The listing builds one solid part. Answer for the finished solid, in the listing's coordinates (mm). A direction names the side the tool comes from. Give positions to 0.01 mm unless a question says otherwise; leave off trailing zeros. Loops run counter-clockwise (first coordinate to the right, second up) from the corner with the lowest first, then second, coordinate; pieces in that order, holes last. Notation, with made-up numbers: (41.25, 85) - (91.25, 85) arc R29 cw to (91.25, 114) - close; hole circle Ø2 at (37.25, 14.5). An arc over 180 degrees is marked (long way). Write each question's results on one line, items separated by ' | '.
from build123d import *

# Parameters (mm, degrees)
SKETCH1_W                                            = 355
SKETCH1_H                                            = 188
BOSS_EXTRUDE1_DEPTH                                  = 3
EDGE_FLANGE1_STRIP_W                                 = 20
EDGE_FLANGE1_STRIP_H                                 = 3
EDGE_FLANGE1_STRIP_CUT_DEPTH                         = 188
EDGE_FLANGE1_DEPTH                                   = 188
SKETCH11_R                                           = 21.5
CUT_EXTRUDE2_DEPTH                                   = 10
CSK_FOR_M4_HEX_SOCKET_COUNTERSUNK_HEAD_S_D           = 4.5
CSK_FOR_M4_HEX_SOCKET_COUNTERSUNK_HEAD_S_DEPTH       = 10
CSK_FOR_M4_HEX_SOCKET_COUNTERSUNK_HEAD_S_CSINK_D     = 9.18
CSK_FOR_M4_HEX_SOCKET_COUNTERSUNK_HEAD_S_CSINK_ANGLE = 90
CSK_FOR_M4_HEX_SOCKET_COUNTERSUNK_HEAD_S_TIP         = 1.351936393
EDGE_FLANGE2_STRIP_W                                 = 20
EDGE_FLANGE2_STRIP_H                                 = 3
EDGE_FLANGE2_STRIP_CUT_DEPTH                         = 188
EDGE_FLANGE2_DEPTH                                   = 188
SKETCH19_W                                           = 210
SKETCH19_H                                           = 48
BOSS_EXTRUDE2_DEPTH                                  = 3
FILLET1_R                                            = 10
EDGE_FLANGE3_STRIP_W                                 = 20
EDGE_FLANGE3_STRIP_H                                 = 3
EDGE_FLANGE3_STRIP_CUT_DEPTH                         = 210
EDGE_FLANGE3_STRIP_2_W                               = 20
EDGE_FLANGE3_STRIP_2_H                               = 3
EDGE_FLANGE3_STRIP_CUT_2_DEPTH                       = 210
EDGE_FLANGE3_DEPTH                                   = 210
EDGE_FLANGE3_BEND_DEPTH                              = 210
SKETCH26_R                                           = 2.1
CUT_EXTRUDE3_DEPTH                                   = 10
SKETCH28_W                                           = 50
SKETCH28_H                                           = 30
CUT_EXTRUDE4_DEPTH                                   = 10
SKETCH29_W                                           = 87
SKETCH29_H                                           = 23.35234987
CUT_EXTRUDE5_DEPTH                                   = 10
FILLET2_R                                            = 10
SKETCH30_R                                           = 2.5
SKETCH30_R_2                                         = 1.57499812
CUT_EXTRUDE6_DEPTH                                   = 10
SKETCH31_R                                           = 2.1
CUT_EXTRUDE7_DEPTH                                   = 236
SKETCH32_R                                           = 2.5
CUT_EXTRUDE8_DEPTH                                   = 10
SKETCH33_R                                           = 2.5
CUT_EXTRUDE9_DEPTH                                   = 10


# Sheet-metal steps are written as plain solids
with BuildPart() as part:
    # Sketch1 → Boss-Extrude1 (new body)
    with BuildSketch(Plane(origin=(0, 0, 0), x_dir=(1, 0, 0), z_dir=(0, 1, 0))):
        Rectangle(SKETCH1_W, SKETCH1_H)
    extrude(amount=BOSS_EXTRUDE1_DEPTH)

    # Edge-Flange1 strip (across the edge) → Edge-Flange1 strip cut (cut)
    with BuildSketch(Plane(origin=(177.5, 3, 94), x_dir=(-1, 0, 0), z_dir=(0, 0, -1))):
        with Locations((-3, -1.5)):
            Rectangle(EDGE_FLANGE1_STRIP_W, EDGE_FLANGE1_STRIP_H)
    extrude(amount=EDGE_FLANGE1_STRIP_CUT_DEPTH, mode=Mode.SUBTRACT)

    # Edge-Flange1 section (across the edge) → Edge-Flange1 (add)
    with BuildSketch(Plane(origin=(177.5, 3, 94), x_dir=(-1, 0, 0), z_dir=(0, 0, -1))):
        with BuildLine():
            Line((0, 4), (0, 52))
            Line((0, 52), (3, 52))
            Line((3, 52), (3, 4))
            ThreePointArc((3, 4), (4.171572875, 1.171572875), (7, 0))
            Line((7, 0), (7, -3))
            ThreePointArc((7, -3), (2.050252532, -0.949747468), (0, 4))
        make_face()
    extrude(amount=EDGE_FLANGE1_DEPTH)

    # Sketch11 → Cut-Extrude2 (cut)
    with BuildSketch(Plane.ZY.offset(-174.5)):
        with Locations(Location((0, 30, 0), (0, 0, 270))):
            Circle(SKETCH11_R)
    extrude(amount=-CUT_EXTRUDE2_DEPTH, mode=Mode.SUBTRACT)

    # CSK for M4 Hex Socket Countersunk Head Screw1
    with Locations(Plane(origin=(177.5, 0, 0), x_dir=(0, 0, -1), z_dir=(1, 0, 0))):
        with Locations((-25, 47.5), (25, 47.5), (25, 12.5), (-25, 12.5)):
            CounterSinkHole(CSK_FOR_M4_HEX_SOCKET_COUNTERSUNK_HEAD_S_D / 2, CSK_FOR_M4_HEX_SOCKET_COUNTERSUNK_HEAD_S_CSINK_D / 2, depth=CSK_FOR_M4_HEX_SOCKET_COUNTERSUNK_HEAD_S_DEPTH, counter_sink_angle=CSK_FOR_M4_HEX_SOCKET_COUNTERSUNK_HEAD_S_CSINK_ANGLE)
            with Locations((0, 0, -(CSK_FOR_M4_HEX_SOCKET_COUNTERSUNK_HEAD_S_DEPTH + CSK_FOR_M4_HEX_SOCKET_COUNTERSUNK_HEAD_S_TIP / 2))):  # 118° drill point
                Cone(0, CSK_FOR_M4_HEX_SOCKET_COUNTERSUNK_HEAD_S_D / 2, CSK_FOR_M4_HEX_SOCKET_COUNTERSUNK_HEAD_S_TIP, mode=Mode.SUBTRACT)

    # Edge-Flange2 strip (across the edge) → Edge-Flange2 strip cut (cut)
    with BuildSketch(Plane(origin=(-177.5, 3, -94), x_dir=(1, 0, 0), z_dir=(0, 0, 1))):
        with Locations((-3, -1.5)):
            Rectangle(EDGE_FLANGE2_STRIP_W, EDGE_FLANGE2_STRIP_H)
    extrude(amount=EDGE_FLANGE2_STRIP_CUT_DEPTH, mode=Mode.SUBTRACT)

    # Edge-Flange2 section (across the edge) → Edge-Flange2 (add)
    with BuildSketch(Plane(origin=(-177.5, 3, -94), x_dir=(1, 0, 0), z_dir=(0, 0, 1))):
        with BuildLine():
            Line((0, 4), (0, 52))
            Line((0, 52), (3, 52))
            Line((3, 52), (3, 4))
            ThreePointArc((3, 4), (4.171572875, 1.171572875), (7, 0))
            Line((7, 0), (7, -3))
            ThreePointArc((7, -3), (2.050252532, -0.949747468), (0, 4))
        make_face()
    extrude(amount=EDGE_FLANGE2_DEPTH)

    # Sketch19 → Boss-Extrude2 (add)
    with BuildSketch(Plane(origin=(0, 3, 0), x_dir=(1, 0, 0), z_dir=(0, 1, 0))):
        with Locations((65.5, 118)):
            Rectangle(SKETCH19_W, SKETCH19_H)
        with Locations((65.5, -118)):
            Rectangle(SKETCH19_W, SKETCH19_H)
    extrude(amount=-BOSS_EXTRUDE2_DEPTH)

    # Fillet1
    fillet1_edges = [part.edges().sort_by_distance(p)[0] for p in [
        (-39.5, 1.5, -94),
        (-39.5, 1.5, 94),
    ]]
    fillet(fillet1_edges, radius=FILLET1_R)

    # Edge-Flange3 strip (across the edge) → Edge-Flange3 strip cut (cut)
    with BuildSketch(Plane(origin=(170.5, 3, -142), x_dir=(0, 0, 1), z_dir=(-1, 0, 0))):
        with Locations((-3, -1.5)):
            Rectangle(EDGE_FLANGE3_STRIP_W, EDGE_FLANGE3_STRIP_H)
    extrude(amount=EDGE_FLANGE3_STRIP_CUT_DEPTH, mode=Mode.SUBTRACT)

    # Edge-Flange3 strip 2 (across the edge) → Edge-Flange3 strip cut 2 (cut)
    with BuildSketch(Plane(origin=(-39.5, 3, 142), x_dir=(0, 0, -1), z_dir=(1, 0, 0))):
        with Locations((-3, -1.5)):
            Rectangle(EDGE_FLANGE3_STRIP_2_W, EDGE_FLANGE3_STRIP_2_H)
    extrude(amount=EDGE_FLANGE3_STRIP_CUT_2_DEPTH, mode=Mode.SUBTRACT)

    # Edge-Flange3 section (across the edge) → Edge-Flange3 (add)
    with BuildSketch(Plane(origin=(170.5, 3, -142), x_dir=(0, 0, 1), z_dir=(-1, 0, 0))):
        with BuildLine():
            Line((0, 4), (0, 27))
            Line((0, 27), (3, 27))
            Line((3, 27), (3, 4))
            ThreePointArc((3, 4), (4.171572875, 1.171572875), (7, 0))
            Line((7, 0), (7, -3))
            ThreePointArc((7, -3), (2.050252532, -0.949747468), (0, 4))
        make_face()
    extrude(amount=EDGE_FLANGE3_DEPTH)

    # Edge-Flange3 section 2 (across the edge) → Edge-Flange3 bend (add)
    with BuildSketch(Plane(origin=(-39.5, 3, 142), x_dir=(0, 0, -1), z_dir=(1, 0, 0))):
        with BuildLine():
            Line((0, 4), (0, 27))
            Line((0, 27), (3, 27))
            Line((3, 27), (3, 4))
            ThreePointArc((3, 4), (4.171572875, 1.171572875), (7, 0))
            Line((7, 0), (7, -3))
            ThreePointArc((7, -3), (2.050252532, -0.949747468), (0, 4))
        make_face()
    extrude(amount=EDGE_FLANGE3_BEND_DEPTH)

    # Sketch26 → Cut-Extrude3 (cut)
    with BuildSketch(Plane(origin=(0, 0, 0), x_dir=(-1, 0, 0), z_dir=(0, -1, 0))):
        with Locations(Location((160.5, -74.75, 0), (0, 0, 90))):
            Circle(SKETCH26_R)
        with Locations(Location((160.5, -84.75, 0), (0, 0, 90))):
            Circle(SKETCH26_R)
        with Locations(Location((100.5, -84.75, 0), (0, 0, 90))):
            Circle(SKETCH26_R)
        with Locations(Location((100.5, -74.75, 0), (0, 0, 90))):
            Circle(SKETCH26_R)
        with Locations(Location((128.5, 74.75, 0), (0, 0, 90))):
            Circle(SKETCH26_R)
        with Locations(Location((128.5, 84.75, 0), (0, 0, 90))):
            Circle(SKETCH26_R)
        with Locations(Location((68.5, 74.75, 0), (0, 0, 90))):
            Circle(SKETCH26_R)
        with Locations(Location((68.5, 84.75, 0), (0, 0, 90))):
            Circle(SKETCH26_R)
    extrude(amount=-CUT_EXTRUDE3_DEPTH, mode=Mode.SUBTRACT)

    # Sketch28 → Cut-Extrude4 (cut)
    with BuildSketch(Plane(origin=(0, 0, -142), x_dir=(-1, 0, 0), z_dir=(0, 0, -1))):
        with Locations((-10.5, 15)):
            Rectangle(SKETCH28_W, SKETCH28_H)
    extrude(amount=-CUT_EXTRUDE4_DEPTH, mode=Mode.SUBTRACT)

    # Sketch29 → Cut-Extrude5 (cut)
    with BuildSketch(Plane.XY.offset(142)):
        with Locations((107, 25.461076577)):
            Rectangle(SKETCH29_W, SKETCH29_H)
    extrude(amount=-CUT_EXTRUDE5_DEPTH, mode=Mode.SUBTRACT)

    # Fillet2
    fillet2_edges = [part.edges().sort_by_distance(p)[0] for p in [
        (63.5, 13.784901642, 140.5),
        (150.5, 13.784901642, 140.5),
    ]]
    fillet(fillet2_edges, radius=FILLET2_R)

    # Sketch30 → Cut-Extrude6 (cut)
    with BuildSketch(Plane(origin=(0, 0, 0), x_dir=(-1, 0, 0), z_dir=(0, -1, 0))):
        with Locations(Location((49.000000561, -50.5, 0), (0, 0, 90))):
            Circle(SKETCH30_R)
        with Locations(Location((49.000000561, 50.5, 0), (0, 0, 90))):
            Circle(SKETCH30_R)
        with Locations(Location((-65.4184, 33.8046, 0), (0, 0, 90))):
            Circle(SKETCH30_R_2)
        with Locations(Location((-155.436, 33.8046, 0), (0, 0, 90))):
            Circle(SKETCH30_R_2)
        with Locations(Location((-155.43961696, 119.9106, 0), (0, 0, 90))):
            Circle(SKETCH30_R_2)
        with Locations(Location((-65.42201696, 119.9614, 0), (0, 0, 90))):
            Circle(SKETCH30_R_2)
    extrude(amount=-CUT_EXTRUDE6_DEPTH, mode=Mode.SUBTRACT)

    # Sketch31 → Cut-Extrude7 (cut)
    with BuildSketch(Plane(origin=(0, 3, 0), x_dir=(1, 0, 0), z_dir=(0, 1, 0))):
        with Locations(Location((-22.75, 113, 0), (0, 0, 270))):
            Circle(SKETCH31_R)
        with Locations(Location((-22.75, 93, 0), (0, 0, 270))):
            Circle(SKETCH31_R)
        with Locations(Location((43.75, 113, 0), (0, 0, 270))):
            Circle(SKETCH31_R)
        with Locations(Location((43.75, 93, 0), (0, 0, 270))):
            Circle(SKETCH31_R)
        with Locations(Location((43.75, 0, 0), (0, 0, 270))):
            Circle(SKETCH31_R)
        with Locations(Location((43.75, -20, 0), (0, 0, 270))):
            Circle(SKETCH31_R)
        with Locations(Location((-3.75, -39, 0), (0, 0, 270))):
            Circle(SKETCH31_R)
        with Locations(Location((24.75, -39, 0), (0, 0, 270))):
            Circle(SKETCH31_R)
        with Locations(Location((-22.75, 0, 0), (0, 0, 270))):
            Circle(SKETCH31_R)
        with Locations(Location((-22.75, -20, 0), (0, 0, 270))):
            Circle(SKETCH31_R)
    extrude(amount=-CUT_EXTRUDE7_DEPTH, mode=Mode.SUBTRACT)

    # Sketch32 → Cut-Extrude8 (cut)
    with BuildSketch(Plane.XY.offset(142)):
        with Locations((-24.5, 18.5)):
            Circle(SKETCH32_R)
        with Locations((1.928571429, 18.5)):
            Circle(SKETCH32_R)
        with Locations((28.357142857, 18.5)):
            Circle(SKETCH32_R)
        with Locations((54.785714286, 18.5)):
            Circle(SKETCH32_R)
        with Locations((160.5, 18.5)):
            Circle(SKETCH32_R)
    extrude(amount=-CUT_EXTRUDE8_DEPTH, mode=Mode.SUBTRACT)

    # Sketch33 → Cut-Extrude9 (cut)
    with BuildSketch(Plane(origin=(0, 0, -142), x_dir=(-1, 0, 0), z_dir=(0, 0, -1))):
        with Locations((-158.5, 18.5)):
            Circle(SKETCH33_R)
        with Locations((-121.3, 18.5)):
            Circle(SKETCH33_R)
        with Locations((-84.1, 18.5)):
            Circle(SKETCH33_R)
        with Locations((-46.9, 18.5)):
            Circle(SKETCH33_R)
        with Locations((27.5, 18.5)):
            Circle(SKETCH33_R)
    extrude(amount=-CUT_EXTRUDE9_DEPTH, mode=Mode.SUBTRACT)


solid = part.part
Item 1: For a pull along X with two mould halves and no side action, classify faces 6 (the face through (-14.5, 14.8, -139.3)), 7 (the face through (66.352, 16.792, 140.479)), 8 (the face through (175.4, 2, 1.3)), 9 (the face through (-177.5, 31, -1)) as released by +X, released by -X, zero draft, split by the parting line, or undercut.
Values found:
face 6: undercut | face 7: undercut | face 8: released by +X | face 9: released by -X
Item 2: A cutting plane is placed at A-A, the plane x = -60. Determine the outline of the cut face in (y, z), plus the area to 3 significant figures.
Values found:
outline: (0, -94) - (3, -94) - (3, 94) - (0, 94) - close | area: 564 mm²
Item 3: Flat-ended cylindrical pins translate along their axes: P1, Ø7, axis at y = 47.5, z = -25, coming from the +X side; P2, Ø4, axis at x = -22.75, z = 0, coming from the +Y side; P3, Ø1.5, axis at x = 101, z = 140.5, coming from the +Y side; P4, Ø5, axis at x = 24.75, z = 39, coming from the +Y side. Find the tip coordinate at first contact, or state that the pin passes through.
Values found:
P1: stops at x = 176.41 | P2: passes through | P3: stops at y = 13.78 | P4: stops at y = 3
Item 4: A cutting plane is placed at B-B, the plane z = 124.5. Determine the outline of the cut face in (x, y).
Values found:
outline: (-39.5, 0) - (170.5, 0) - (170.5, 3) - (-39.5, 3) - close
Item 5: For faces 1 (the face through (-174.5, 31, -1)), 2 (the face through (170.5, 2.8, 123.2)), 3 (the face through (-142, 1, 94)), 4 (the face through (-142, 1, -94)), 5 (the face through (170.5, 2.8, -123.2)), determine the directions among +Z, -Z, +X, -X, +Y, -Y from which every point of the face is accessible in a straight line to the end or side of a thin tool.
Values found:
face 1: +Z, -Z, +Y | face 2: +Z, +X, +Y, -Y | face 3: +Z, -X, +Y, -Y | face 4: -Z, -X, +Y, -Y | face 5: -Z, +X, +Y, -Y
Item 6: Find the intervals of material crossed by line 1 along X through (y, z) = (1, -113); line 2 along X through (y, z) = (10, -12.5); line 3 along Z through (x, y) = (-17, 25), in increasing order. Write a range as [from, to].
Values found:
line 1: x = [-39.5, -24.85], [-20.65, 41.65], [45.85, 170.5] | line 2: x = [-177.5, -174.5], [174.5, 177.5] | line 3: z = [-142, -139], [139, 142]
